```python
from build123d import *

# Parameters (mm, degrees)
SKETCH1_W                 = 4
SKETCH1_H                 = 12
SKETCH1_W_2               = 8
BOSS_EXTRUDE1_DEPTH       = 5
F_4_0MM_DOWEL_HOLE1_D     = 4
F_4_0MM_DOWEL_HOLE1_DEPTH = 10
F_4_0MM_DOWEL_HOLE1_TIP   = 1.201721238
CUT_EXTRUDE1_START        = -12
SKETCH5_W                 = 3
SKETCH5_H                 = 3
CUT_EXTRUDE1_DEPTH        = 12


with BuildPart() as part:
    # Sketch1 → Revolve1 (revolve)
    with BuildSketch(Plane.XY):
        with Locations((6, 6)):
            Rectangle(SKETCH1_W, SKETCH1_H)
        with Locations((4, 18)):
            Rectangle(SKETCH1_W_2, SKETCH1_H)
    revolve(axis=Axis((0, 0, 0), (0, 1, 0)))

    # Sketch2 → Boss-Extrude1 (add)
    with BuildSketch(Plane(origin=(0, 24, 0), x_dir=(1, 0, 0), z_dir=(0, 1, 0))):
        Polygon((6.92820323, 0), (3.464101615, 6), (-3.464101615, 6), (-6.92820323, 0), (-3.464101615, -6), (3.464101615, -6), align=None)
    extrude(amount=BOSS_EXTRUDE1_DEPTH)

    # Ø4.0mm Dowel Hole1
    with Locations(Plane(origin=(0, 29, 0), x_dir=(1, 0, 0), z_dir=(0, 1, 0))):
        with Locations((0, 0)):
            Hole(F_4_0MM_DOWEL_HOLE1_D / 2, depth=F_4_0MM_DOWEL_HOLE1_DEPTH)
            with Locations((0, 0, -(F_4_0MM_DOWEL_HOLE1_DEPTH + F_4_0MM_DOWEL_HOLE1_TIP / 2))):  # 118° drill point
                Cone(0, F_4_0MM_DOWEL_HOLE1_D / 2, F_4_0MM_DOWEL_HOLE1_TIP, mode=Mode.SUBTRACT)

    # Sketch5 → Cut-Extrude1 (cut)
    with BuildSketch(Plane.XZ.offset(CUT_EXTRUDE1_START)):
        with Locations((4, 0)):
            Rectangle(SKETCH5_W, SKETCH5_H)
    extrude(amount=CUT_EXTRUDE1_DEPTH, mode=Mode.SUBTRACT)


solid = part.part
```
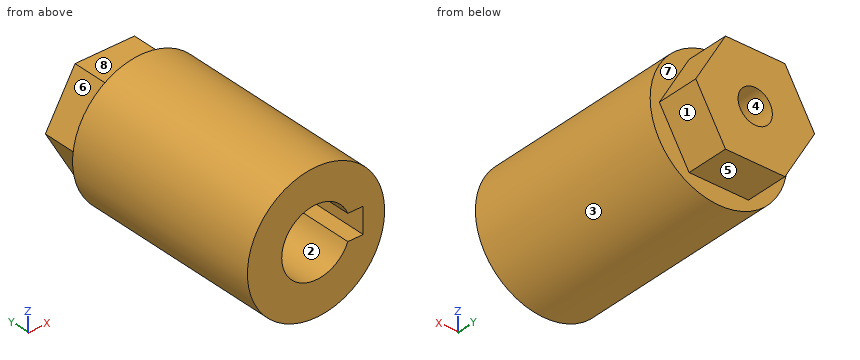
Check sheet for the modelled part. Datum: model origin and axes. Units: mm. Face numbers are marked on the shaded views. A direction names the side the tool comes from. Round coordinates to 2 decimals unless told otherwise and drop trailing zeros. Loops run counter-clockwise (first coordinate to the right, second up) from the corner with the lowest first, then second, coordinate; pieces in that order, holes last. Notation, with made-up numbers: (14.5, -10.5) -> (68.5, -10.5) arc R18 ccw to (68.5, 3.5) -> close; hole circle Ø10 at (13, -26.5). An arc over 180 degrees is marked (long way). Write item = value, one per line. Start each with the question number.
1) Release check for a two-part mould opening along Z. For the marked faces 1, 2, 3 and 4 record: released by +Z, released by -Z, zero draft, split by the parting line, or undercut.
2) Sectioned sample at D-D, the plane z = -5.5. Record the cut outline in (x, y), plus the area to 3 significant figures.
3) Thickness scan on probe 1 along Z at (x, y) = (0, 4.5); probe 2 along Y at (x, z) = (-0.25, 3.5); probe 3 along Z at (x, y) = (1, 9.75). Record the ranges inside material, lowest first.
4) Sectioned sample at B-B, the plane z = -2.5. Record the cut outline in (x, y).
5) Gauge pin test, flat ends, axial feed: pin 1 Ø0.9 at (x, y) = (4, 6) entering from -Z; pin 2 Ø2.5 at (x, z) = (0.5, 2) entering from -Y; pin 3 Ø0.9 at (x, y) = (4.5, 3) entering from +Z. Record the tip position at first contact, or that the pin passes through.
6) Set-up check for the marked faces 5, 6, 7 and 8: record each of +Z, -Z, +X, -X, +Y, -Y from which the full face is reachable in a straight line by a thin tool's end or side.
7) Sectioned sample at A-A, the plane y = 8. Record the cut outline in (x, z).
8) Sectioned sample at C-C, the plane y = 15.25. Record the cut outline in (x, z), plus the area to 3 significant figures.
Results are:
q1.face_1 = released by -Z
q1.face_2 = undercut
q1.face_3 = split by the parting line
q1.face_4 = undercut
q2.outline = (-5.81, 0) -> (5.81, 0) -> (5.81, 24) -> (3.75, 24) -> (3.75, 29) -> (-3.75, 29) -> (-3.75, 24) -> (-5.81, 24) -> close
q2.area = 316 mm^2
q3.probe_1 = -8 to -4, 4 to 8
q3.probe_2 = 12 to 29
q3.probe_3 = -7.94 to -3.87, 3.87 to 7.94
q4.outline = (-7.6, 0) -> (-3.12, 0) -> (-3.12, 12) -> (3.12, 12) -> (3.12, 0) -> (7.6, 0) -> (7.6, 24) -> (5.48, 24) -> (5.48, 29) -> (-5.48, 29) -> (-5.48, 24) -> (-7.6, 24) -> close
q5.pin_1 = -7.17
q5.pin_2 = 12
q5.pin_3 = 6.9
q6.face_5 = -Z, +X, -X, +Y
q6.face_6 = +Z, -X, +Y
q6.face_7 = +Y
q6.face_8 = +Z, +X, -X, +Y
q7.outline = circle Ø16 at (0, 0); hole (3.71, -1.5) -> (5.5, -1.5) -> (5.5, 1.5) -> (3.71, 1.5) arc R4 ccw (long way) to start
q8.outline = circle Ø16 at (0, 0)
q8.area = 201 mm^2
